Design review of the part built by this model. Coordinates are the model's own, in mm. Coordinates: 2 decimals unless noted, no trailing zeros. Loops run counter-clockwise (first coordinate to the right, second up) from the corner with the lowest first, then second, coordinate; pieces in that order, holes last. Notation, with made-up numbers: (32.5, 75) -> (64.5, 75) arc R31 ccw to (64.5, 106) -> close; hole circle Ø8 at (44, -36.75). An arc over 180 degrees is marked (long way). Use one line per item in the form item = value. Start each with the question number.
1. For pin 1 (5 mm diameter, centred on x = 86.56, y = 40, fed in from +Z); pin 2 (5 mm diameter, centred on x = -43.44, y = -30, fed in from +Z); pin 3 (10 mm diameter, centred on x = 31.5, y = -18, fed in from -Z); pin 4 (12 mm diameter, centred on x = -29, y = 27, fed in from +Z), all flat-tipped, find the tip position at first contact; note any pin that passes through.
2. Consider section A-A (y = 30). State the section outline as (x, z) points.
3. Consider section D-D (y = -40). State the section outline as (x, z) points, then the cut area to 3 significant figures.
4. Consider section B-B (z = 0.65). State the section outline as (x, y) points.
5. Wall thickness on line 1 (X direction, y = 30, z = 0.7); line 2 (Y direction, x = 87.5, z = 0.8); line 3 (Z direction, x = -27.5, y = -32): over which ranges is each line inside the solid? List them lowest first. Write a range as from..to.
6. Consider section C-C (x = 82). State the section outline as (y, z) points, then the cut area to 3 significant figures.
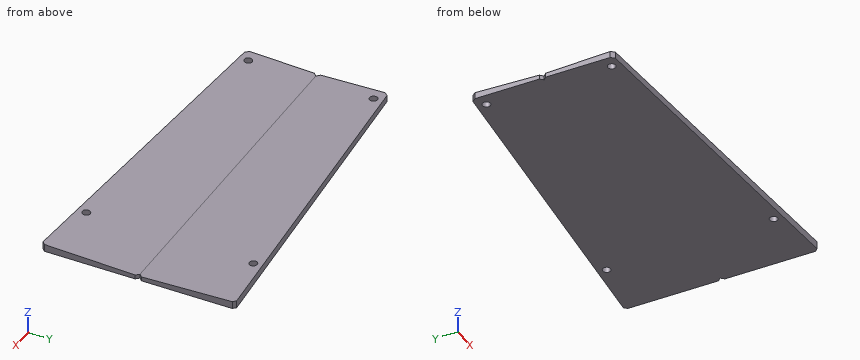
from build123d import *

# Parameters (mm, degrees)
ESQUISSE1_R      = 1.9
EXTRUSION1_DEPTH = 2
D_POUILLE1_ANGLE = 2
CHANFREIN1_SIZE  = 1.5
CHANFREIN1_SIZE2 = 1.398361753
CHANFREIN2_SIZE  = 1.5
CHANFREIN3_SIZE  = 1.5
CHANFREIN4_SIZE  = 1.5
CHANFREIN4_SIZE2 = 1.627601385


with BuildPart() as part:
    # Esquisse1 → Extrusion1 (new body)
    with BuildSketch(Plane.XY):
        Polygon((-49.438888889, 0), (115.561111111, 0), (115.561111111, 46.5), (-49.438888889, 34), align=None)
        with Locations((86.561111111, 40)):
            Circle(ESQUISSE1_R, mode=Mode.SUBTRACT)
        with Locations((-43.438888889, 30)):
            Circle(ESQUISSE1_R, mode=Mode.SUBTRACT)
    extrude(amount=EXTRUSION1_DEPTH)

    # Dépouille1
    d_pouille1_faces = [part.faces().sort_by_distance(p)[0] for p in [
        (37.385342989, 20.236326134, 2),
    ]]
    draft(d_pouille1_faces, Plane(origin=(-49.438888889, 0, 2), x_dir=(0, 0, -1), z_dir=(0, -1, 0)), D_POUILLE1_ANGLE)

    # Chanfrein1
    chanfrein1_edges = [part.edges().sort_by_distance(p)[0] for p in [
        (115.561111111, 46.5, 1.811907891),
    ]]
    chanfrein1_side = [part.faces().sort_by_distance(p)[0] for p in [
        (115.561111111, 25.487728403, 1.445025544),
    ]]
    chamfer(chanfrein1_edges, length=CHANFREIN1_SIZE, length2=CHANFREIN1_SIZE2, reference=chanfrein1_side[0])

    # Chanfrein2
    chanfrein2_edges = [part.edges().sort_by_distance(p)[0] for p in [
        (115.561111111, 0, 1),
    ]]
    chamfer(chanfrein2_edges, length=CHANFREIN2_SIZE)

    # Chanfrein3
    chanfrein3_edges = [part.edges().sort_by_distance(p)[0] for p in [
        (-49.438888889, 0, 1),
    ]]
    chamfer(chanfrein3_edges, length=CHANFREIN3_SIZE)

    # Chanfrein4
    chanfrein4_edges = [part.edges().sort_by_distance(p)[0] for p in [
        (-49.438888889, 34, 1.593653081),
    ]]
    chanfrein4_side = [part.faces().sort_by_distance(p)[0] for p in [
        (34.097619228, 40.328523342, 1.704151534),
    ]]
    chamfer(chanfrein4_edges, length=CHANFREIN4_SIZE, length2=CHANFREIN4_SIZE2, reference=chanfrein4_side[0])

    # Symétrie1: part across plane


with BuildPart() as part_1:
    add(part.part)
    add(part.part.mirror(Plane(origin=(-49.438888889, 0, 2), x_dir=(0, 0, 1), z_dir=(0, 1, 0))))


solid = part_1.part
Geometry check:
q1.pin_1 = 3.48
q1.pin_2 = 3.13
q1.pin_3 = 0
q1.pin_4 = 3.15
q2.outline = (-49.44, 0) -> (-45.34, 0) -> (-45.34, 3.05) -> (-49.44, 3.05) -> close; (-41.54, 0) -> (115.56, 0) -> (115.56, 3.05) -> (-41.54, 3.05) -> close
q3.outline = (29.76, 0) -> (84.66, 0) -> (84.66, 3.4) -> (29.76, 3.4) -> close; (88.46, 0) -> (115.56, 0) -> (115.56, 3.4) -> (88.46, 3.4) -> close
q3.area = 279 mm²
q4.outline = (-49.44, -32.37) -> (-47.94, -34.11) -> (114.17, -46.39) -> (115.56, -45) -> (115.56, -1.5) -> (114.06, 0) -> (115.56, 1.5) -> (115.56, 45) -> (114.17, 46.39) -> (-47.94, 34.11) -> (-49.44, 32.37) -> (-49.44, 1.5) -> (-47.94, 0) -> (-49.44, -1.5) -> close; hole circle Ø3.8 at (-43.44, -30); hole circle Ø3.8 at (-43.44, 30); hole circle Ø3.8 at (86.56, -40); hole circle Ø3.8 at (86.56, 40)
q5.line_1 = -49.44..-45.34, -41.54..115.56
q5.line_2 = -44.37..-41.65, -38.35..38.35, 41.65..44.37
q5.line_3 = 0..3.12
q6.outline = (-43.96, 0) -> (43.96, 0) -> (43.96, 3.54) -> (0, 2) -> (-43.96, 3.54) -> close
q6.area = 243 mm²
